from build123d import *

# Parameters (mm, degrees)
F1_DEPTH = 76.2
F2_DEPTH = 254
F3_DEPTH = 25.4


with BuildPart() as f1:
    # F0 (on Front) → F1 (new body)
    with BuildSketch(Plane.XZ):
        Polygon((-15.184847, -13.14384), (-25.345129, -13.14384), (-25.345129, -15.692936), (25.454871, -15.692936), (25.454871, -13.14384), (15.294871, -13.14384), (12.754871, -13.14384), (-12.756689, -13.14384), align=None)
    extrude(amount=F1_DEPTH)

    # F0 (on Front) → F2 (join)
    with BuildSketch(Plane.XZ):
        Polygon((-15.184847, -13.14384), (-25.345129, -13.14384), (-25.345129, -15.692936), (25.454871, -15.692936), (25.454871, -13.14384), (15.294871, -13.14384), (12.754871, -13.14384), (-12.756689, -13.14384), align=None)
    extrude(amount=-F2_DEPTH)

    # F0 (on Front) → F3 (join)
    with BuildSketch(Plane.XZ):
        with BuildLine():
            Line((-15.184847, 1.1065), (-15.184847, -13.14384))
            Line((-15.184847, -13.14384), (-12.756689, -13.14384))
            Line((-12.756689, -13.14384), (-12.699554, 0.13098))
            ThreePointArc((-12.699554, 0.13098), (-8.941194, 9.095144), (0.054989, 12.776202))
            Line((0.054989, 12.776202), (0.109531, 12.775968))
            ThreePointArc((0.109531, 12.775968), (9.054432, 9.036995), (12.754871, 0.076085))
            Line((12.754871, 0.076085), (12.754871, -13.14384))
            Line((12.754871, -13.14384), (15.294871, -13.14384))
            Line((15.294871, -13.14384), (15.294871, 1.084637))
            ThreePointArc((15.294871, 1.084637), (11.594432, 10.045547), (2.649531, 13.784519))
            Line((2.649531, 13.784519), (-2.430187, 13.806382))
            ThreePointArc((-2.430187, 13.806382), (-11.445757, 10.10606), (-15.184847, 1.1065))
        make_face()
    extrude(amount=-F3_DEPTH)


solid = f1.part
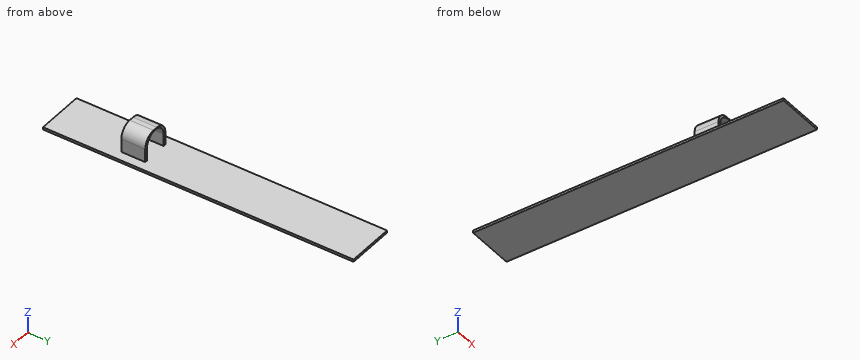
Geometry: final body of the model. Coordinates: model frame, mm. Give positions to 0.01 mm unless a question says otherwise; leave off trailing zeros. Loops run counter-clockwise (first coordinate to the right, second up) from the corner with the lowest first, then second, coordinate; pieces in that order, holes last. Notation, with made-up numbers: (31.5, 23.25) - (85.5, 23.25) arc R7 ccw to (85.5, 30.25) - close; hole circle Ø5 at (-15.75, -10.75). An arc over 180 degrees is marked (long way). Answer as CSV lines item,"result". Start each with the question number.
1. Section B-B, the plane z = 9.75. Return loops of the section in (x, y).
2. Ray query, L1, parallel to Y at x = 6, z = 11.5; L2, parallel to Z at x = 15.5, y = 29; L3, parallel to X at y = 12, z = -2.75. Return the intervals inside material, ascending.
3. Pin query (flat end, axial travel): P1, Ø4, axis at x = -11, y = 104, coming from the +Z side; P2, Ø4.5, axis at y = 15, z = -8.5, coming from the +X side; P3, Ø6.5, axis at y = 18, z = -4, coming from the -X side. Return the tip coordinate at first contact, or that it passes through.
4. Section C-C, the plane y = 48.5. Return loops of the section in (x, z), plus the area to 3 significant figures.
5. Section A-A, the plane z = -5.5. Return loops of the section in (x, y).
Answers:
1,outline,"(-11.79, 0) - (-8.23, 0) - (-8.23, 25.4) - (-11.79, 25.4) - close; (8.28, 0) - (11.88, 0) - (11.88, 25.4) - (8.28, 25.4) - close"
2,L1,"y = 0 to 25.4"
2,L2,"z = -15.69 to -13.14"
2,L3,"x = -15.18 to -12.71, 12.75 to 15.29"
3,P1,"stops at z = -13.14"
3,P2,"stops at x = 15.29"
3,P3,"stops at x = -15.18"
4,outline,"(-25.35, -15.69) - (25.45, -15.69) - (25.45, -13.14) - (-25.35, -13.14) - close"
4,area,"129 mm2"
5,outline,"(-15.18, 0) - (-12.72, 0) - (-12.72, 25.4) - (-15.18, 25.4) - close; (12.75, 0) - (15.29, 0) - (15.29, 25.4) - (12.75, 25.4) - close"
